```python
from build123d import *

# Parameters (mm, degrees)
SKETCH1_W                       = 60
SKETCH1_H                       = 15
BOSS_EXTRUDE1_DEPTH             = 5
SKETCH2_W                       = 37
SKETCH2_H                       = 15
BOSS_EXTRUDE2_DEPTH             = 10
FILLET1_R                       = 5
SKETCH3_W                       = 29
SKETCH3_H                       = 30
BOSS_EXTRUDE3_DEPTH             = 5
FILLET2_R                       = 5
BOSS_EXTRUDE6_REACH             = 26
SKETCH8_W                       = 6
SKETCH8_H                       = 30
BOSS_EXTRUDE6_DIRECTION_2_REACH = 39
SKETCH7_W                       = 6
SKETCH7_H                       = 22
CUT_EXTRUDE3_DEPTH              = 11
REVOLVE1_ANGLE                  = 90


with BuildPart() as part:
    # Sketch1 → Boss-Extrude1 (new body)
    with BuildSketch(Plane.XY):
        Rectangle(SKETCH1_W, SKETCH1_H)
    extrude(amount=BOSS_EXTRUDE1_DEPTH)

    # Sketch2 → Boss-Extrude2 (add)
    with BuildSketch(Plane.ZY.offset(30)):
        with Locations((-13.5, 0)):
            Rectangle(SKETCH2_W, SKETCH2_H)
    extrude(amount=BOSS_EXTRUDE2_DEPTH)

    # Fillet1
    fillet1_edges = [part.edges().sort_by_distance(p)[0] for p in [
        (-40, 0, 5),
    ]]
    fillet(fillet1_edges, radius=FILLET1_R)

    # Sketch3 → Boss-Extrude3 (add)
    with BuildSketch(Plane(origin=(30, 0, 0), x_dir=(0, 0, -1), z_dir=(1, 0, 0))):
        with Locations((-14.5, 7.5)):
            Rectangle(SKETCH3_W, SKETCH3_H)
    extrude(amount=BOSS_EXTRUDE3_DEPTH)

    # Fillet2
    fillet2_edges = [part.edges().sort_by_distance(p)[0] for p in [
        (35, 7.5, 0),
    ]]
    fillet(fillet2_edges, radius=FILLET2_R)

    # Boss-Extrude6: up to this face of the body (flat: up to its plane)
    boss_extrude6_end = Plane(part.part.faces().sort_by_distance((32.5, 7.5, 29))[0])
    # Sketch8 → Boss-Extrude6 (add, up to the picked face)
    with BuildSketch(Plane.XY.offset(5), mode=Mode.PRIVATE) as boss_extrude6_sk1:
        with Locations((27, 7.5)):
            Rectangle(SKETCH8_W, SKETCH8_H)
    boss_extrude6_tool1 = split(extrude(boss_extrude6_sk1.sketch, amount=BOSS_EXTRUDE6_REACH, mode=Mode.PRIVATE), bisect_by=boss_extrude6_end, keep=Keep.BOTH, mode=Mode.PRIVATE)
    add(boss_extrude6_tool1.solids().sort_by(Axis((27, 7.5, 5), (0, 0, 1)))[0])

    # Boss-Extrude6 direction 2: up to this face of the body (flat: up to its plane)
    boss_extrude6_direction_2_end = Plane(part.part.faces().sort_by_distance((0, 0, 0))[0])
    # Sketch8 → Boss-Extrude6 direction 2 (add, up to the picked face)
    with BuildSketch(Plane.XY.offset(5), mode=Mode.PRIVATE) as boss_extrude6_direction_2_sk1:
        with Locations((27, 7.5)):
            Rectangle(SKETCH8_W, SKETCH8_H)
    boss_extrude6_direction_2_tool1 = split(extrude(boss_extrude6_direction_2_sk1.sketch, amount=-BOSS_EXTRUDE6_DIRECTION_2_REACH, mode=Mode.PRIVATE), bisect_by=boss_extrude6_direction_2_end, keep=Keep.BOTH, mode=Mode.PRIVATE)
    add(boss_extrude6_direction_2_tool1.solids().sort_by(Axis((27, 7.5, 5), (0, 0, -1)))[0])

    # Sketch7 → Cut-Extrude3 (cut)
    with BuildSketch(Plane.XZ.offset(7.5)):
        with Locations((30, 16)):
            Rectangle(SKETCH7_W, SKETCH7_H)
        with Locations((-35, -16)):
            Rectangle(SKETCH7_W, SKETCH7_H)
    extrude(amount=-CUT_EXTRUDE3_DEPTH, mode=Mode.SUBTRACT)

    # Sketch9 → Revolve1 (revolve)
    with BuildSketch(Plane.ZY.offset(-24)):
        with BuildLine():
            Line((15.5, 15.75), (29, 15.75))
            ThreePointArc((29, 15.75), (22.25, 22.5), (15.5, 15.75))
        make_face()
        with BuildLine():
            ThreePointArc((13.5, 15.75), (6.75, 22.5), (0, 15.75))
            Line((0, 15.75), (13.5, 15.75))
        make_face()
    revolve(axis=Axis((24, 15.75, 0), (0, 0, 1)), revolution_arc=REVOLVE1_ANGLE)


with BuildPart() as body_2:
    # Mirror1: mirrored copy
    add(part.part.mirror(Plane(origin=(-40, 7.5, -32), x_dir=(1, 0, 0), z_dir=(0, 0, 1))))


solid = body_2.part
```
Input: part model. Units: mm. Frame: model coordinates. A direction names the side the tool comes from. Round coordinates to 2 decimals unless told otherwise and drop trailing zeros. Write each loop counter-clockwise with the first axis right and the second up, starting at its lowest first coordinate (ties: lowest second). Pieces come first, ordered by that corner, then holes. Notation, with made-up numbers: M -26.75,46 L 26.25,46 A33 cw 26.25,75 Z; hole C 16,47.25 d5. An arc over 180 degrees is marked long. Write each question's results on one line, items separated by ' | '.
Q1. Access query for faces 1 (the face through (0, 1, -64)), 2 (the face through (24, 21, -65)), 3 (the face through (-35, -2, -37)), 4 (the face through (21, 15.75, -71)). Directions: +Z, -Z, +X, -X, +Y, -Y. A direction counts if a zero-diameter tool reaches every point of the face in a straight line with its end or side. Return the directions, or none.
Results:
face 1: +Z, +X, +Y, -Y | face 2: +Z, -X, +Y | face 3: -Y | face 4: +Z, -Z, -X
Q2. Section query A-A (y = 1). Return loops of the section in (x, z).
Results:
outline: M -40,-64 A5 ccw -35,-69 L 24,-69 L 24,-93 L 35,-93 L 35,-69 A5 ccw 30,-64 L -30,-64 L -30,-32 L -40,-32 Z; hole M -38,-59 L -32,-59 L -32,-37 L -38,-37 Z; hole M 27,-91 L 33,-91 L 33,-69 L 27,-69 Z
Q3. Section query B-B (z = -43). Return loops of the section in (x, y), and give its area (3 significant figures).
Results:
outline: M -40,-7.5 L -38,-7.5 L -38,3.5 L -32,3.5 L -32,-7.5 L -30,-7.5 L -30,7.5 L -40,7.5 Z | area: 84.0 mm^2
Q4. Draft query along Z for faces 5 (the face through (29, 7, -93)), 6 (the face through (30, 3.5, -80)), 7 (the face through (34, 8, -66)), 8 (the face through (24, 21, -92)). Return one class per face: released by +Z, released by -Z, zero draft, split by the parting line, or undercut.
Results:
face 5: released by -Z | face 6: undercut | face 7: released by +Z | face 8: zero draft
Q5. Line query: line 1 along X through (y, z) = (-6, -46); line 2 along X through (y, z) = (0.75, -89); line 3 along Z through (x, y) = (-12, 1.5). Output: solid intervals per line, ascending.
Results:
line 1: x = -40 to -38, -32 to -30 | line 2: x = 24 to 27, 33 to 35 | line 3: z = -69 to -64
Q6. Section query C-C (x = -33.5). Return loops of the section in (y, z).
Results:
outline: M -7.5,-69 L 7.5,-69 L 7.5,-32 L -7.5,-32 L -7.5,-37 L 3.5,-37 L 3.5,-59 L -7.5,-59 Z
Q7. Pin query (flat end, axial travel): P1, Ø2, axis at y = 19, z = -88, coming from the -X side; P2, Ø2, axis at x = 20, z = -70.5, coming from the -Y side; P3, Ø15, axis at x = 7, y = 3.5, coming from the +Z side. Return the tip coordinate at first contact, or that it passes through.
Results:
P1: stops at x = 17.81 | P2: stops at y = 15.75 | P3: stops at z = -64
Q8. Section query D-D (y = 19.25). Return loops of the section in (x, z), and give its area (3 significant figures).
Results:
outline: M 24,-93 L 35,-93 L 35,-69 A5 ccw 30,-64 L 24,-64 L 24,-64.98 A5.77 ccw 24,-76.52 L 24,-80.48 A5.77 ccw 24,-92.02 Z | area: 418 mm^2
